Input: part model. Units: mm. Frame: model coordinates. Face numbers are marked on the shaded views. A direction names the side the tool comes from. Coordinates: 2 decimals unless noted, no trailing zeros. Loops run counter-clockwise (first coordinate to the right, second up) from the corner with the lowest first, then second, coordinate; pieces in that order, holes last.
(1) Set-up query: the marked faces 1, 2, 3, 4 and 5. Return all of +Z, -Z, +X, -X, +Y, -Y with unobstructed straight access to the full face (end or side cutting, diameter ignored); none if empty.
(2) Contact query for flat-ended pins moving along their axis: P1, Ø2.5, axis at y = -24.5, z = 2.5, coming from the +X side; P2, Ø9, axis at x = -38.5, y = -26.5, coming from the +Z side; P3, Ø4, axis at x = -37.5, z = -1, coming from the +Y side; P4, Ø5, axis at x = 37, y = 25, coming from the -Z side. Output: stop coordinate, or through.
(3) Section A-A, the plane z = -4.75. Return loops of the section in (x, y), then the cut area to 3 significant figures.
(4) Line query: L1, parallel to Y at x = -37, z = -7.15; L2, parallel to Y at x = -35.5, z = 1.5. Output: solid intervals per line, ascending.
```python
from build123d import *

# Parameters (mm, degrees)
F0_W     = 83
F0_H     = 59
F1_DEPTH = 7.5
F2_R     = 1.5
F3_DEPTH = 15.001
F4_R     = 4.5
F5_W     = 8
F5_H     = 8
F6_DEPTH = 14


with BuildPart() as f1:
    # F0 (on Top) → F1 (new body, symmetric)
    with BuildSketch(Plane.XY):
        Rectangle(F0_W, F0_H)
    extrude(amount=F1_DEPTH, both=True)

    # F2 (on face) → F3 (cut, through all)
    with BuildSketch(Plane.XY.offset(7.5)):
        with Locations((-37, 25)):
            Circle(F2_R)
        with Locations((37, 25)):
            Circle(F2_R)
        with Locations((-37, -25)):
            Circle(F2_R)
        with Locations((37, -25)):
            Circle(F2_R)
    extrude(amount=-F3_DEPTH, mode=Mode.SUBTRACT)

    # F4
    f4_edges = [f1.edges().sort_by_distance(p)[0] for p in [
        (-41.5, 29.5, 0),
        (-41.5, -29.5, 0),
        (41.5, -29.5, 0),
        (41.5, 29.5, 0),
    ]]
    fillet(f4_edges, radius=F4_R)

    # F5 (on face) → F6 (cut)
    with BuildSketch(Plane.XY.offset(7.5)):
        with Locations((-37.5, 25.5)):
            Rectangle(F5_W, F5_H)
        with Locations((37.5, 25.5)):
            Rectangle(F5_W, F5_H)
        with Locations((-37.5, -25.5)):
            Rectangle(F5_W, F5_H)
        with Locations((37.5, -25.5)):
            Rectangle(F5_W, F5_H)
    extrude(amount=-F6_DEPTH, mode=Mode.SUBTRACT)


solid = f1.part
```
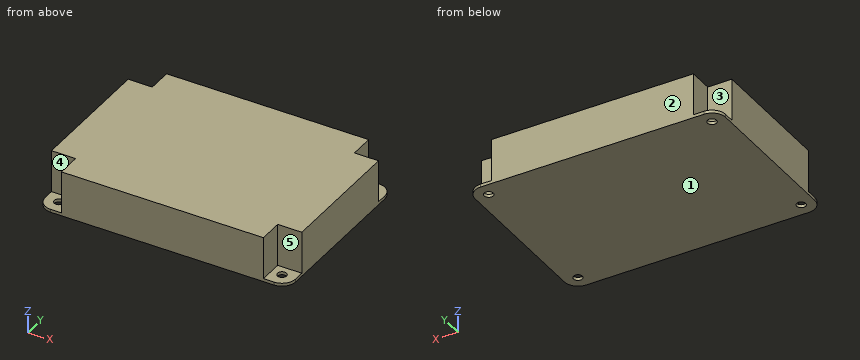
Report:
1. face 1: -Z, +X, -X, +Y, -Y
1. face 2: +Z, -Z, +X, -X, +Y
1. face 3: +Z, -X, +Y
1. face 4: +Z, -X, -Y
1. face 5: +Z, +X, -Y
2. P1: stops at x = 33.5
2. P2: stops at z = -6.5
2. P3: stops at y = 21.5
2. P4: stops at z = -7.5
3. outline: (-41.5, -21.5) - (-33.5, -21.5) - (-33.5, -29.5) - (33.5, -29.5) - (33.5, -21.5) - (41.5, -21.5) - (41.5, 21.5) - (33.5, 21.5) - (33.5, 29.5) - (-33.5, 29.5) - (-33.5, 21.5) - (-41.5, 21.5) - close
3. area: 4,640 mm2
4. L1: y = -29.5 to -26.5, -23.5 to 23.5, 26.5 to 29.5
4. L2: y = -21.5 to 21.5
